Design review of the part built by this model. Coordinates are the model's own, in mm. A direction names the side the tool comes from. Give positions to 0.01 mm unless a question says otherwise; leave off trailing zeros. Write each loop counter-clockwise with the first axis right and the second up, starting at its lowest first coordinate (ties: lowest second). Pieces come first, ordered by that corner, then holes. Notation, with made-up numbers: M 3.25,33.5 L 16.25,33.5 A15 ccw 16.25,40.5 Z; hole C 0,69.25 d11. An arc over 180 degrees is marked long. Answer in a Markdown table with one row per item.
```python
from build123d import *

# Parameters (mm, degrees)
F0_W     = 104
F0_H     = 104
F0_W_2   = 43.8093654811
F0_H_2   = 16.4691451937
F1_DEPTH = 100
F2_DEPTH = 5
F3_T     = -2.5
F4_R     = 15
F5_DEPTH = 25


with BuildPart() as f1:
    # F0 (on Front) → F1 (new body)
    with BuildSketch(Plane.XZ):
        Rectangle(F0_W, F0_H)
        Rectangle(F0_W_2, F0_H_2, mode=Mode.SUBTRACT)
    extrude(amount=F1_DEPTH)

    # F0 (on Front) → F2 (join)
    with BuildSketch(Plane.XZ):
        Rectangle(F0_W_2, F0_H_2)
    extrude(amount=F2_DEPTH)

    # F3
    f3_openings = [f1.faces().sort_by_distance(p)[0] for p in [
        (0, -52.5, -8.234573),
        (21.904683, -52.5, 0),
        (0, -52.5, 8.234573),
        (-21.904683, -52.5, 0),
        (0, -5, 0),
    ]]
    offset(amount=F3_T, openings=f3_openings)

    # F4 (on face) → F5 (cut)
    with BuildSketch(Plane(origin=(0, 0, 0), x_dir=(-1, 0, 0), z_dir=(0, 1, 0))):
        Circle(F4_R)
    extrude(amount=-F5_DEPTH, mode=Mode.SUBTRACT)


solid = f1.part
```
1) Add section C-C (x = -23.5). Write out the cut boundary in (y, z).
Geometry says:
| item | result |
|---|---|
| outline | M -100,-52 L 0,-52 L 0,52 L -100,52 Z; hole M -97.5,-49.5 L -2.5,-49.5 L -2.5,49.5 L -97.5,49.5 Z |
2) The part is to be moulded in two halves that separate along Z. For faces 1 (the face through (52, -49, -1)), 2 (the face through (-12, -2.5, 12)), 3 (the face through (-1, -49, -52)), say which applies: released by +Z, released by -Z, zero draft, split by the parting line, or undercut.
Geometry says:
| item | result |
|---|---|
| face 1 | zero draft |
| face 2 | undercut |
| face 3 | released by -Z |
3) Add section D-D (z = 0). Write out the cut boundary in (x, y).
Geometry says:
| item | result |
|---|---|
| outline | M -52,-100 L -21.9,-100 L -21.9,-97.5 L -49.5,-97.5 L -49.5,-2.5 L -15,-2.5 L -15,0 L -52,0 Z; M 15,-2.5 L 49.5,-2.5 L 49.5,-97.5 L 21.9,-97.5 L 21.9,-100 L 52,-100 L 52,0 L 15,0 Z |
4) Add section B-B (z = 45.5). Write out the cut boundary in (x, y), and give its area (3 significant figures).
Geometry says:
| item | result |
|---|---|
| outline | M -52,-100 L 52,-100 L 52,0 L -52,0 Z; hole M -49.5,-97.5 L 49.5,-97.5 L 49.5,-2.5 L -49.5,-2.5 Z |
| area | 995 mm^2 |
5) To check wall thickness, follow probe 1 along Z at (x, y) = (-8.5, -38); probe 2 along Z at (x, y) = (0, -1.4); probe 3 along Y at (x, z) = (6.5, 28). State the ranges of each line that lie inside material, in increasing order. Write a range as [from, to].
Geometry says:
| item | result |
|---|---|
| probe 1 | [-52, -49.5], [49.5, 52] |
| probe 2 | [-52, -15], [15, 52] |
| probe 3 | [-100, -97.5], [-2.5, 0] |
6) Insertion check: P1, Ø18, axis at x = 0, z = 0, coming from the -Y side. The pin has a flat end and moves straight along its axis. Give the tip position at first contact, or say it passes through.
Geometry says:
| item | result |
|---|---|
| P1 | y = -100 |
7) Add section A-A (x = 0). Write out the cut boundary in (y, z).
Geometry says:
| item | result |
|---|---|
| outline | M -100,-52 L 0,-52 L 0,-15 L -2.5,-15 L -2.5,-49.5 L -97.5,-49.5 L -97.5,-8.23 L -100,-8.23 Z; M -100,8.23 L -97.5,8.23 L -97.5,49.5 L -2.5,49.5 L -2.5,15 L 0,15 L 0,52 L -100,52 Z |
8) For faces 4 (the face through (14.985, -1.232, 0.66)), 5 (the face through (-12, 0, 12)), 6 (the face through (-49.5, -49, -1)), list the 3-axis set-ups (+Z, -Z, +X, -X, +Y, -Y) from which the entire face can be reached by the end or side of a thin tool; tool diameter is ignored.
Geometry says:
| item | result |
|---|---|
| face 4 | +Y |
| face 5 | +Z, -Z, +X, -X, +Y |
| face 6 | none |
